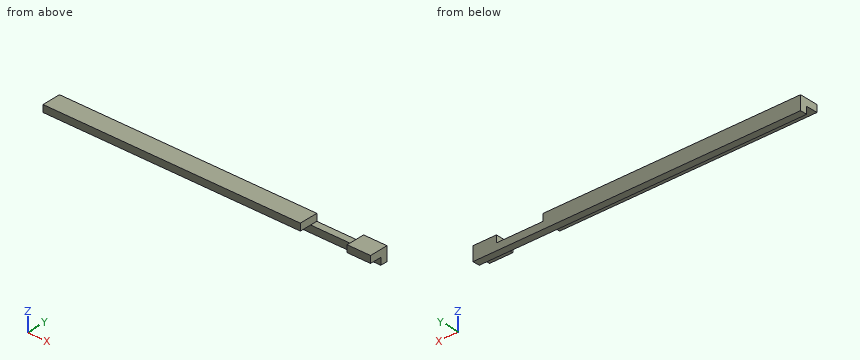
```python
from build123d import *

# Parameters (mm, degrees)
SKETCH1_W           = 140
SKETCH1_H           = 8
BOSS_EXTRUDE1_DEPTH = 8
SKETCH2_W           = 3
SKETCH2_H           = 5
SKETCH2_W_2         = 2
SKETCH2_H_2         = 8
CUT_EXTRUDE1_DEPTH  = 140
SKETCH4_W           = 20
SKETCH4_H           = 8
CUT_EXTRUDE2_DEPTH  = 3


with BuildPart() as part:
    # Sketch1 → Boss-Extrude1 (new body)
    with BuildSketch(Plane(origin=(0, 0, 0), x_dir=(1, 0, 0), z_dir=(0, 1, 0))):
        Rectangle(SKETCH1_W, SKETCH1_H)
    extrude(amount=BOSS_EXTRUDE1_DEPTH)

    # Sketch2 → Cut-Extrude1 (cut)
    with BuildSketch(Plane(origin=(70, 0, 0), x_dir=(0, 0, -1), z_dir=(1, 0, 0))):
        with Locations((2.5, 2.5)):
            Rectangle(SKETCH2_W, SKETCH2_H)
        with Locations((-3, 4)):
            Rectangle(SKETCH2_W_2, SKETCH2_H_2)
    extrude(amount=-CUT_EXTRUDE1_DEPTH, mode=Mode.SUBTRACT)

    # Sketch4 → Cut-Extrude2 (cut)
    with BuildSketch(Plane.XY.offset(2)):
        with Locations((50, 4)):
            Rectangle(SKETCH4_W, SKETCH4_H)
    extrude(amount=-CUT_EXTRUDE2_DEPTH, mode=Mode.SUBTRACT)


solid = part.part
```
Could you check a few things on this model? Use its own coordinates, in mm. Coordinates: 2 decimals unless noted, no trailing zeros. Loops run counter-clockwise (first coordinate to the right, second up) from the corner with the lowest first, then second, coordinate; pieces in that order, holes last. Notation, with made-up numbers: M -8,19.5 L -3,19.5 A24 ccw -3,55.5 Z; hole C 3.5,21.25 d11. An arc over 180 degrees is marked long. Put each result on its own line as item: value. Start each with the question number.
(1) Suppose I cut it at A-A on z = 0.4. Please give me the cut outline in (x, y).
(2) Will these pins go through, and if not, where does the flat tip stop? P1, Ø1, axis at x = 45.5, z = -2.5, coming from the -Y side; P2, Ø1.5, axis at x = -34.5, y = 2.5, coming from the -Z side; P3, Ø2.5, axis at x = 52, y = 6, coming from the +Z side.
(3) I need wall thicknesses on line 1 (X direction, y = 7.5, z = 1.2); line 2 (Y direction, x = 16, z = -1.15); line 3 (Z direction, x = -1.5, y = 3.75). Which ranges of each line are inside material? Lowest first, please. Write a range as from..to.
(4) Suppose I cut it at B-B on x = 25. Please give me the cut outline in (y, z).
(5) Suppose I cut it at C-C on x = 55.5. Please give me the cut outline in (y, z).
Solutions:
1. outline: M -70,0 L 40,0 L 40,8 L -70,8 Z; M 60,0 L 70,0 L 70,8 L 60,8 Z
2. P1: stops at y = 5
2. P2: stops at z = -1
2. P3: stops at z = -1
3. line 1: x = -70..40, 60..70
3. line 2: y = 5..8
3. line 3: z = -1..2
4. outline: M 0,-1 L 5,-1 L 5,-4 L 8,-4 L 8,2 L 0,2 Z
5. outline: M 5,-4 L 8,-4 L 8,-1 L 5,-1 Z
